from build123d import *

# Parameters (mm, degrees)
SKETCH1_R           = 10.16
BOSS_EXTRUDE1_DEPTH = 15.24
BOSS_EXTRUDE2_DEPTH = 6.35
SKETCH3_R           = 12.7
BOSS_EXTRUDE3_DEPTH = 12.7
SKETCH4_R           = 7.62
CUT_EXTRUDE1_DEPTH  = 41.387863689


with BuildPart() as part:
    # Sketch1 → Boss-Extrude1 (new body)
    with BuildSketch(Plane(origin=(0, 0, 0), x_dir=(1, 0, 0), z_dir=(0, 1, 0))):
        with Locations(Location((0, 0, 0), (0, 0, 90))):
            Circle(SKETCH1_R)
    extrude(amount=BOSS_EXTRUDE1_DEPTH)

    # Sketch2 → Boss-Extrude2 (add)
    with BuildSketch(Plane.XZ):
        Polygon((-13.97, -8.065583261), (0, -16.131166521), (13.97, -8.065583261), (13.97, 8.065583261), (0, 16.131166521), (-13.97, 8.065583261), align=None)
    extrude(amount=BOSS_EXTRUDE2_DEPTH)

    # Sketch3 → Boss-Extrude3 (add)
    with BuildSketch(Plane.XZ.offset(6.35)):
        with Locations(Location((0, 0, 0), (0, 0, 270))):
            Circle(SKETCH3_R)
    extrude(amount=BOSS_EXTRUDE3_DEPTH)

    # Sketch4 → Cut-Extrude1 (cut, through all)
    with BuildSketch(Plane(origin=(0, 15.24, 0), x_dir=(1, 0, 0), z_dir=(0, 1, 0))):
        with Locations(Location((0, 0, 0), (0, 0, 270))):
            Circle(SKETCH4_R)
    extrude(amount=-CUT_EXTRUDE1_DEPTH, mode=Mode.SUBTRACT)


solid = part.part
Model file for the job. Use its own axes, mm. A direction names the side the tool comes from. Give positions to 0.01 mm unless a question says otherwise; leave off trailing zeros. Order: outer loops, then holes, each group sorted by start corner. A loop starts at its lowest first (then second) coordinate and runs counter-clockwise, first axis right, second up. Notation, with made-up numbers: (41, 40) - (46, 40) arc R7 ccw to (46, 53) - close; hole circle Ø8 at (88, -8.75). An arc over 180 degrees is marked (long way). Write item = value, one per line. Start each with the question number.
1. Two-plate mould, pull along Z, no slides. Class faces 4 (the flat face through (-13.97, -3, 0)), 5 (the cylindrical face through (7.555, -1.665, -0.992)), 6 (the flat face through (-6.887, -3.131, 12.155)), 7 (the flat face through (6.887, -3.131, -12.155)): pulls with the +Z half, pulls with the -Z half, needs draft (parallel to the pull), parting line crosses it, or undercut.
2. Cut at C-C, the plane y = -1.5. List the corners of the cut face in (x, z), and give its area (3 significant figures).
3. Probe line 1 along X through (y, z) = (-8, 0); line 2 along X through (y, z) = (2.5, 0); line 3 along Y through (x, z) = (-2, -13). List the from-to ranges inside material, lowest first.
4. Cut at D-D, the plane z = 9.5. List the corners of the cut face in (x, y).
5. Cut at A-A, the plane x = 7. List the corners of the cut face in (y, z), and give its area (3 significant figures).
6. Which spindle directions (+Z, -Z, +X, -X, +Y, -Y) get a long thin tool onto all of the face, cutting with end or side? Do faces 1 (the flat face through (-5, -6.35, -12)), 2 (the flat face through (-8, 15.24, -1)), 3 (the flat face through (0, 0, -11)). Say none if no direction does.
7. Drop flat-ended pins along their axis: P1, Ø2, axis at x = 5.5, y = 2.5, coming from the -Z side; P2, Ø1.5, axis at x = -8.5, y = 9.5, coming from the +Z side; P3, Ø6, axis at y = 9, z = 9, coming from the +X side. Give the stop position or say it passes through.
8. Cut at B-B, the plane z = 0. List the corners of the cut face in (x, y).
Taken from the geometry:
q1.face_4 = needs draft
q1.face_5 = undercut
q1.face_6 = pulls with the +Z half
q1.face_7 = pulls with the -Z half
q2.outline = (-13.97, -8.07) - (0, -16.13) - (13.97, -8.07) - (13.97, 8.07) - (0, 16.13) - (-13.97, 8.07) - close; hole circle Ø15.24 at (0, 0)
q2.area = 494 mm²
q3.line_1 = -12.7 to -7.62, 7.62 to 12.7
q3.line_2 = -10.16 to -7.62, 7.62 to 10.16
q3.line_3 = -6.35 to 0
q4.outline = (-11.49, -6.35) - (-8.43, -6.35) - (-8.43, -19.05) - (8.43, -19.05) - (8.43, -6.35) - (11.49, -6.35) - (11.49, 0) - (3.6, 0) - (3.6, 15.24) - (-3.6, 15.24) - (-3.6, 0) - (-11.49, 0) - close
q5.outline = (-19.05, -10.6) - (-6.35, -10.6) - (-6.35, -12.09) - (0, -12.09) - (0, -7.36) - (15.24, -7.36) - (15.24, -3.01) - (-19.05, -3.01) - close; (-19.05, 3.01) - (15.24, 3.01) - (15.24, 7.36) - (0, 7.36) - (0, 12.09) - (-6.35, 12.09) - (-6.35, 10.6) - (-19.05, 10.6) - close
q5.area = 441 mm²
q6.face_1 = -Y
q6.face_2 = +Z, -Z, +X, -X, +Y
q6.face_3 = +Y
q7.P1 = -9.11
q7.P2 = 6.57
q7.P3 = 8.2
q8.outline = (-13.97, -6.35) - (-12.7, -6.35) - (-12.7, -19.05) - (-7.62, -19.05) - (-7.62, 15.24) - (-10.16, 15.24) - (-10.16, 0) - (-13.97, 0) - close; (7.62, -19.05) - (12.7, -19.05) - (12.7, -6.35) - (13.97, -6.35) - (13.97, 0) - (10.16, 0) - (10.16, 15.24) - (7.62, 15.24) - close
